Check sheet for the drawn part. Datum: minimum x, y, z corner. Units: mm. A direction names the side the tool comes from. Coordinates: 2 decimals unless noted, no trailing zeros. Write each loop counter-clockwise with the first axis right and the second up, starting at its lowest first coordinate (ties: lowest second). Pieces come first, ordered by that corner, then holes. Notation, with made-up numbers: (-5, 72.25) - (52, 72.25) arc R31 cw to (52, 99.25) - close; hole circle Ø9 at (-10, 65.25). An arc over 180 degrees is marked (long way). Write each question's results on one line, items separated by ' | '.
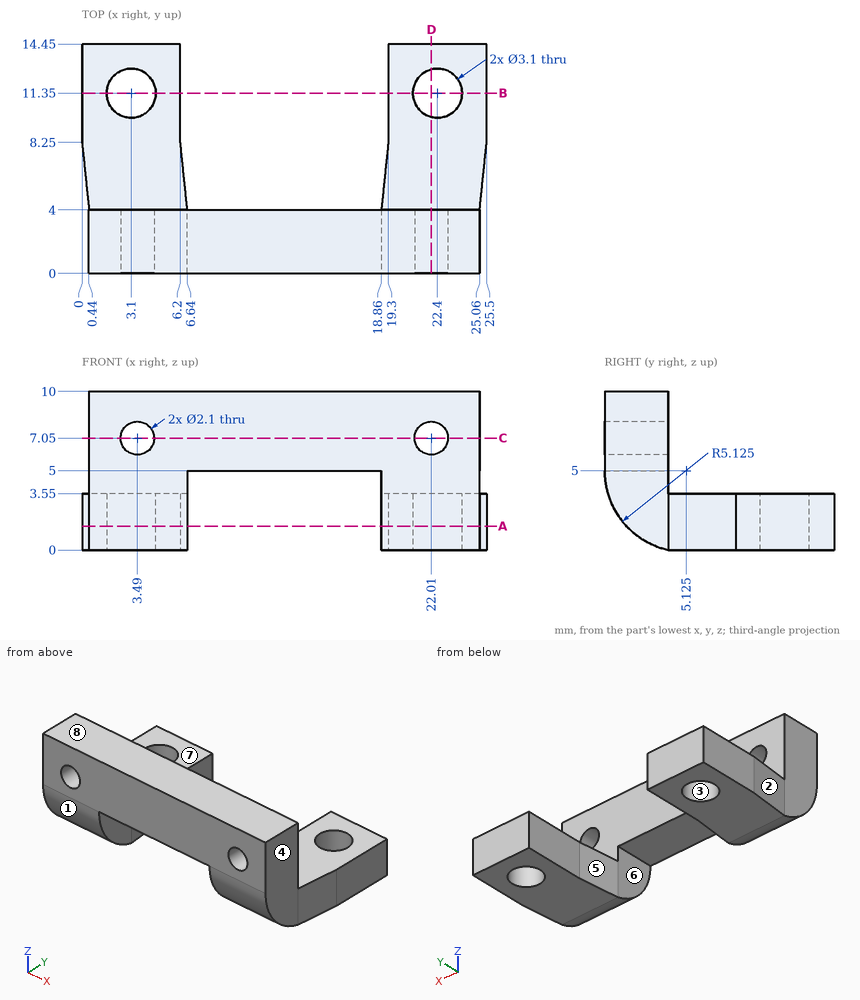
1. Draft check along X on the marked faces 1, 2 and 3. Enter one of: pulls with the +X half, pulls with the -X half, needs draft (parallel to the pull), parting line crosses it, or undercut.
Values follow:
face 1: needs draft | face 2: pulls with the -X half | face 3: undercut
2. Material ranges on L1, parallel to X at y = 11.35, z = 1.9; L2, parallel to X at y = 2.6, z = 7.05; L3, parallel to X at y = 12.5, z = 3.25, recorded low to high. Write a range as [from, to].
Values follow:
L1: x = [0, 1.55], [4.65, 6.2], [19.3, 20.85], [23.95, 25.5] | L2: x = [0.44, 2.44], [4.54, 20.96], [23.06, 25.06] | L3: x = [0, 2.06], [4.14, 6.2], [19.3, 21.36], [23.44, 25.5]
3. Sectioned sample at C-C (z = 7.05). Record the cut outline in (x, y).
Values follow:
outline: (0.44, 0) - (2.44, 0) - (2.44, 4) - (0.44, 4) - close; (4.54, 0) - (20.96, 0) - (20.96, 4) - (4.54, 4) - close; (23.06, 0) - (25.06, 0) - (25.06, 4) - (23.06, 4) - close
4. Sectioned sample at B-B (y = 11.35). Record the cut outline in (x, z), then the cut area to 3 significant figures.
Values follow:
outline: (0, 0) - (1.55, 0) - (1.55, 3.55) - (0, 3.55) - close; (4.65, 0) - (6.2, 0) - (6.2, 3.55) - (4.65, 3.55) - close; (19.3, 0) - (20.85, 0) - (20.85, 3.55) - (19.3, 3.55) - close; (23.95, 0) - (25.5, 0) - (25.5, 3.55) - (23.95, 3.55) - close | area: 22.0 mm^2
5. Go/stop test with flat-tipped pins: pin 1 (1.2 mm diameter, centred on y = 3, z = 3, fed in from -X); pin 2 (4 mm diameter, centred on y = 5.5, z = 5, fed in from -X); pin 3 (3.5 mm diameter, centred on x = 3.1, y = 11.35, fed in from +Z). Record where each tip stops, or that it passes through.
Values follow:
pin 1: stops at x = 0.44 | pin 2: stops at x = 0.14 | pin 3: stops at z = 3.55
6. Access from +Z, -Z, +X, -X, +Y, -Y to the whole of each face (thin tool, end or side, straight path). Record for the marked faces 4, 5, 6, 7 and 8.
Values follow:
face 4: +Z, -Z, +X, -Y | face 5: +Z, -Z, +Y | face 6: -Z, +Y, -Y | face 7: +Z, +X, -X, +Y | face 8: +Z, +X, -X, +Y, -Y
7. Sectioned sample at A-A (z = 1.5). Record the cut outline in (x, y).
Values follow:
outline: (0, 8.25) - (0.44, 4) - (0.44, 1.38) - (6.64, 1.38) - (6.64, 4) - (6.2, 8.25) - (6.2, 14.45) - (0, 14.45) - close; (18.86, 1.38) - (25.06, 1.38) - (25.06, 4) - (25.5, 8.25) - (25.5, 14.45) - (19.3, 14.45) - (19.3, 8.25) - (18.86, 4) - close; hole circle Ø3.1 at (3.1, 11.35); hole circle Ø3.1 at (22.4, 11.35)
8. Sectioned sample at D-D (x = 22.01). Record the cut outline in (y, z) (3 decimals).
Values follow:
outline: (0, 5) arc R5.125 ccw to (4, 0) - (9.85, 0) - (9.85, 3.55) - (4, 3.55) - (4, 6) - (0, 6) - close; (0, 8.1) - (4, 8.1) - (4, 10) - (0, 10) - close; (12.85, 0) - (14.45, 0) - (14.45, 3.55) - (12.85, 3.55) - close
